from build123d import *

# Parameters (mm, degrees)
SKETCH_1_R      = 2
EXTRUDE_1_DEPTH = 4


with BuildPart() as part:
    # 草图1 → 凸台-拉伸1 (new body)
    with BuildSketch(Plane.XY):
        with BuildLine():
            Line((-21, 23.478713764), (-21, 25))
            Line((-21, 25), (-46, 25))
            Line((-46, 25), (-46, -25))
            Line((-46, -25), (-21, -25))
            Line((-21, -25), (-21, -23.478713764))
            ThreePointArc((-21, -23.478713764), (-31.5, 0), (-21, 23.478713764))
        make_face()
        with Locations((-40, 20)):
            Circle(SKETCH_1_R, mode=Mode.SUBTRACT)
        with Locations((-40, -20)):
            Circle(SKETCH_1_R, mode=Mode.SUBTRACT)
    extrude(amount=EXTRUDE_1_DEPTH)


solid = part.part
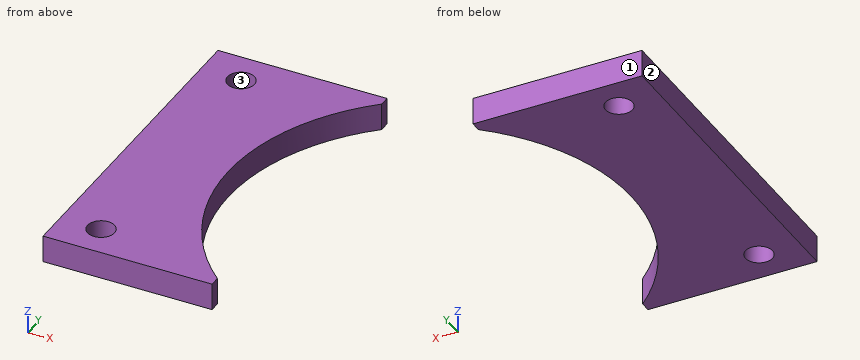
Part model, mm, in its own coordinate system. Face numbers are marked on the shaded views. Give positions to 0.01 mm unless a question says otherwise; leave off trailing zeros. Loops run counter-clockwise (first coordinate to the right, second up) from the corner with the lowest first, then second, coordinate; pieces in that order, holes last.
(1) Pin check, flat tips, straight feed: pin 1 (10 mm diameter, centred on x = -24.5, y = -2, fed in from -Z); pin 2 (8 mm diameter, centred on x = -38.5, y = -17, fed in from -Z). Stop position of each tip, or through.
Return value:
pin 1: passes through
pin 2: stops at z = 0
(2) Drill centre lines: line 1 along Y through (x, z) = (-40, 2.75); line 2 along Y through (x, z) = (-41, 1.3); line 3 along Y through (x, z) = (-25, 0.7). Where is each one in solid material? Low to high.
Return value:
line 1: y = -25 to -22, -18 to 18, 22 to 25
line 2: y = -25 to -21.73, -18.27 to 18.27, 21.73 to 25
line 3: y = -25 to -19.16, 19.16 to 25
(3) Band-saw the part on B-B (x = -29.5). Write the cut outline in (y, z), and give its area (3 significant figures).
Return value:
outline: (-25, 0) - (-11.05, 0) - (-11.05, 4) - (-25, 4) - close; (11.05, 0) - (25, 0) - (25, 4) - (11.05, 4) - close
area: 112 mm2
(4) Band-saw the part on C-C (z = 1.55). Write the cut outline in (x, y), and give its area (3 significant figures).
Return value:
outline: (-46, -25) - (-21, -25) - (-21, -23.48) arc R31.5 cw to (-21, 23.48) - (-21, 25) - (-46, 25) - close; hole circle Ø4 at (-40, -20); hole circle Ø4 at (-40, 20)
area: 883 mm2
(5) Band-saw the part on D-D (y = 20). Write the cut outline in (x, z).
Return value:
outline: (-46, 0) - (-42, 0) - (-42, 4) - (-46, 4) - close; (-38, 0) - (-24.34, 0) - (-24.34, 4) - (-38, 4) - close
(6) Band-saw the part on A-A (x = -40). Write the cut outline in (y, z), and give its area (3 significant figures).
Return value:
outline: (-25, 0) - (-22, 0) - (-22, 4) - (-25, 4) - close; (-18, 0) - (18, 0) - (18, 4) - (-18, 4) - close; (22, 0) - (25, 0) - (25, 4) - (22, 4) - close
area: 168 mm2
(7) Pull direction Y, two halves, no side cores. Call the marked faces 1, 2 and 3: pulls with the +Y half, pulls with the -Y half, needs draft (parallel to the pull), parting line crosses it, or undercut.
Return value:
face 1: pulls with the +Y half
face 2: needs draft
face 3: undercut
